Input: part model. Units: mm. Frame: model coordinates. Round coordinates to 2 decimals unless told otherwise and drop trailing zeros. Write each loop counter-clockwise with the first axis right and the second up, starting at its lowest first coordinate (ties: lowest second). Pieces come first, ordered by that corner, then holes. Notation, with made-up numbers: M 11,13 L 32,13 A22 ccw 32,47 Z; hole C 60.5,3 d8. An arc over 180 degrees is marked long. Answer as CSV lines item,"result". Start each with the question number.
```python
from build123d import *

# Parameters (mm, degrees)
F0_R     = 32.4231
F0_W     = 25.4
F0_H     = 3.175
F0_R_2   = 4.7625
F1_DEPTH = 3.175


with BuildPart() as f1:
    # F0 (on Top) → F1 (new body)
    with BuildSketch(Plane.XY):
        Circle(F0_R)
        with Locations((0, -17.18679)):
            Rectangle(F0_W, F0_H, mode=Mode.SUBTRACT)
        with Locations((-16.21155, 0)):
            Circle(F0_R_2, mode=Mode.SUBTRACT)
        with Locations((16.21155, 0)):
            Circle(F0_R_2, mode=Mode.SUBTRACT)
    extrude(amount=F1_DEPTH)


solid = f1.part
```
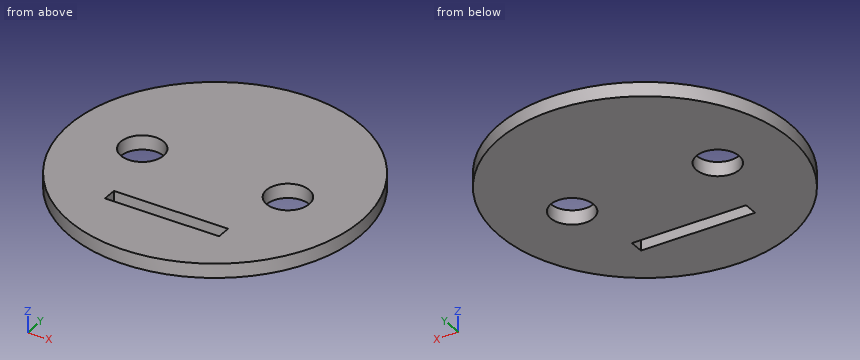
Item 1: Cut plane A-A, the plane x = 0. Return loops of the section in (y, z) (3 decimals), plus the area to 3 significant figures.
Item 2: Line query: line 1 (X direction, y = -16, z = 1.75); line 2 (Y direction, x = 6, z = 0.5); line 3 (Y direction, x = 17.5, z = 1.2). Output: solid intervals per line, ascending. Write a range as [from, to].
Item 3: Cut plane B-B, the plane z = 2.6. Return loops of the section in (x, y) (1 decimal), plus the area to 3 significant figures.
Item 4: Cut plane C-C, the plane y = 0. Return loops of the section in (x, z) (3 decimals), plus the area to 3 significant figures.
Item 5: Pin query (flat end, axial travel): pin 1 Ø15 at (x, y) = (16.21, 0) entering from -Z; pin 2 Ø1.5 at (y, z) = (24.5, 1) entering from +X; pin 3 Ø1.5 at (x, z) = (-10, 0.5) entering from -Y. Return the tip coordinate at first contact, or that it passes through.
Item 6: Cut plane D-D, the plane x = 9. Return loops of the section in (y, z) (3 decimals).
Results list:
1,outline,"M -32.423,0 L -18.774,0 L -18.774,3.175 L -32.423,3.175 Z; M -15.599,0 L 32.423,0 L 32.423,3.175 L -15.599,3.175 Z"
1,area,"196 mm²"
2,line 1,"[-28.2, -12.7], [12.7, 28.2]"
2,line 2,"[-31.86, -18.77], [-15.6, 31.86]"
2,line 3,"[-27.29, -4.58], [4.58, 27.29]"
3,outline,"C 0,0 d64.8; hole C -16.2,0 d9.5; hole M -12.7,-18.8 L 12.7,-18.8 L 12.7,-15.6 L -12.7,-15.6 Z; hole C 16.2,0 d9.5"
3,area,"3,080 mm²"
4,outline,"M -32.423,0 L -20.974,0 L -20.974,3.175 L -32.423,3.175 Z; M -11.449,0 L 11.449,0 L 11.449,3.175 L -11.449,3.175 Z; M 20.974,0 L 32.423,0 L 32.423,3.175 L 20.974,3.175 Z"
4,area,"145 mm²"
5,pin 1,"z = 0"
5,pin 2,"x = 22.07"
5,pin 3,"y = -31.08"
6,outline,"M -31.149,0 L -18.774,0 L -18.774,3.175 L -31.149,3.175 Z; M -15.599,0 L 31.149,0 L 31.149,3.175 L -15.599,3.175 Z"
